from build123d import *

# Parameters (mm, degrees)
SKETCH_W           = 20
SKETCH_H           = 20
PAD_DEPTH          = 2
SKETCH001_W        = 21.291687
SKETCH001_H        = 2
PAD001_DEPTH       = 20
POCKET_DEPTH       = 43
PAD002_DEPTH       = 1
PAD003_DEPTH       = 1
SKETCH004_R        = 2.5
POCKET001_DEPTH    = 5
SKETCH005_R        = 2.5
POCKET002_DEPTH    = 5
POCKET003_DEPTH    = 5
POCKET003_FACE1_W  = 20
POCKET003_FACE1_H  = 2
POCKET004_DEPTH    = 1.846
POCKET005_DEPTH    = 2.202
POCKET006_DEPTH    = 5
SKETCH006_W        = 32.068451
SKETCH006_H        = 15.041733
POCKET007_DEPTH    = 5
POCKET008_DEPTH    = 2
POCKET009_DEPTH    = 2
POCKET010_DEPTH    = 0.5
POCKET011_DEPTH    = 0.5
POCKET011_FACE18_W = 2.5141439852
POCKET011_FACE18_H = 1
POCKET012_DEPTH    = 5
POCKET012_FACE12_W = 1
POCKET012_FACE12_H = 2.5
POCKET013_DEPTH    = 5
POCKET014_DEPTH    = 0.5
POCKET014_FACE5_W  = 1
POCKET014_FACE5_H  = 0.5
POCKET015_DEPTH    = 5
POCKET016_DEPTH    = 0.5
POCKET016_FACE4_W  = 0.5
POCKET016_FACE4_H  = 1
POCKET017_DEPTH    = 7.2
PAD004_DEPTH       = 3.202
PAD005_DEPTH       = 4.846


with BuildPart() as part:
    # Sketch → Pad (new body)
    with BuildSketch(Plane.XY):
        with Locations((318.7276667125, 240.4208782875)):
            Rectangle(SKETCH_W, SKETCH_H)
    extrude(amount=-PAD_DEPTH)

    # Sketch001 (on Face6 of Pad) → Pad001 (join)
    with BuildSketch(Plane(origin=(0, 0, -2), x_dir=(1, 0, 0), z_dir=(0, 0, -1))):
        with Locations((319.1250915, -231.419662)):
            Rectangle(SKETCH001_W, SKETCH001_H)
    extrude(amount=PAD001_DEPTH)

    # Pad001 Face5 → Pocket (cut)
    with BuildSketch(Plane(origin=(325.2175581813, 231.4103392408, -2), x_dir=(0, 1, 0), z_dir=(0, 0, 1))):
        Polygon((1.0093227592, 16.7383101813), (-0.9906772408, 16.7383101813), (-0.9906772408, -4.5533768187), (1.0093227592, -4.5533768187), (1.0093227592, -3.5101085312), (-0.9894609532, -3.5101085312), (-0.9894609532, 16.4898914688), (1.0093227592, 16.4898914688), align=None)
    extrude(amount=-POCKET_DEPTH, mode=Mode.SUBTRACT)

    # Sketch002 (on Face7 of Pocket) → Pad002 (join)
    with BuildSketch(Plane(origin=(308.7276667125, 0, 0), x_dir=(0, -1, 0), z_dir=(-1, 0, 0))):
        Polygon((-250.405853, 0), (-230.420715, -22), (-230.420715, 0), align=None)
    extrude(amount=-PAD002_DEPTH)

    # Sketch003 (on Face2 of Pad002) → Pad003 (join)
    with BuildSketch(Plane.YZ.offset(328.7276667125)):
        Polygon((230.420883, 0.034144), (250.420822, 0.034144), (230.420883, -22.000002), align=None)
    extrude(amount=-PAD003_DEPTH)

    # Sketch004 (on Face6 of Pad003) → Pocket001 (cut)
    with BuildSketch(Plane(origin=(0, 232.419662, 0), x_dir=(-1, 0, 0), z_dir=(0, 1, 0))):
        with Locations((-318.723811, -11.999702)):
            Circle(SKETCH004_R)
    extrude(amount=-POCKET001_DEPTH, mode=Mode.SUBTRACT)

    # Sketch005 (on Face5 of Pocket001) → Pocket002 (cut)
    with BuildSketch(Plane(origin=(0, 0, -2), x_dir=(1, 0, 0), z_dir=(0, 0, -1))):
        with Locations((318.727692, -240.420898)):
            Circle(SKETCH005_R)
    extrude(amount=-POCKET002_DEPTH, mode=Mode.SUBTRACT)

    # Pocket002 Face19 → Pocket003 (cut)
    with BuildSketch(Plane(origin=(327.7276667125, 240.4131065518, 0.0170764125), x_dir=(0, 1, 0), z_dir=(-1, 0, 0))):
        Polygon((-9.9922235518, -0.0170675875), (10.0077154482, -0.0170675875), (9.976723645, 0.0170764125), (-9.9922235518, 0.0170764125), align=None)
    extrude(amount=-POCKET003_DEPTH, mode=Mode.SUBTRACT)

    # Pocket003 Face1 → Pocket004 (cut)
    with BuildSketch(Plane(origin=(318.7276667125, 250.4208782875, -1), x_dir=(1, 0, 0), z_dir=(0, 1, 0))):
        Rectangle(POCKET003_FACE1_W, POCKET003_FACE1_H)
    extrude(amount=-POCKET004_DEPTH, mode=Mode.SUBTRACT)

    # Pocket004 Face7 → Pocket005 (cut)
    with BuildSketch(Plane(origin=(318.7276662811, 231.4202701891, -22), x_dir=(0, -1, 0), z_dir=(0, 0, -1))):
        Polygon((-0.9993918109, 9.9999995686), (-0.9993918109, -10.0000004314), (0.9993853738, -10.0000004314), (0.9993853738, -9.0000004314), (0.9993871891, -9.0000004314), (0.9993871891, -10.0000004314), (0.9993919016, -10.0000004314), (0.9993919016, 9.9999995686), align=None)
    extrude(amount=-POCKET005_DEPTH, mode=Mode.SUBTRACT)

    # Pocket005 Face11 → Pocket006 (cut)
    with BuildSketch(Plane(origin=(309.7276667125, 230.4207966437, -10.9999550626), x_dir=(0, -1, 0), z_dir=(1, 0, 0))):
        Polygon((-8.16439e-05, 10.9998651876), (-8.16439e-05, 8.7980449374), (-8.16439e-05, -10.9999550626), (8.16437e-05, -10.9999550626), (8.16437e-05, 11.0000449374), align=None)
    extrude(amount=-POCKET006_DEPTH, mode=Mode.SUBTRACT)

    # Sketch006 (on Face7 of Pocket006) → Pocket007 (cut)
    with BuildSketch(Plane(origin=(0, 0, -19.798), x_dir=(1, 0, 0), z_dir=(0, 0, -1))):
        with Locations((318.3954625, -232.1317065)):
            Rectangle(SKETCH006_W, SKETCH006_H)
    extrude(amount=POCKET007_DEPTH, mode=Mode.SUBTRACT)

    # Pocket007 Face15 → Pocket008 (cut)
    with BuildSketch(Plane(origin=(318.7273379116, 231.4203047573, -19.798), x_dir=(0, -1, 0), z_dir=(0, 0, -1))):
        Polygon((-0.9993572427, 8.9996711991), (-0.9993572427, -10.0003288009), (0.9994264698, -10.0003288009), (0.9994264698, 9.9996711991), (-1.0007408734, 9.9996711991), (-1.0007408734, 8.9996711991), align=None)
    extrude(amount=-POCKET008_DEPTH, mode=Mode.SUBTRACT)

    # Pocket008 Face3 → Pocket009 (cut)
    with BuildSketch(Plane(origin=(318.7276667125, 248.5748782875, -1), x_dir=(1, 0, 0), z_dir=(0, 1, 0))):
        Polygon((10, -1), (10, 1), (-9, 1), (-10, 1), (-10, -1), align=None)
    extrude(amount=-POCKET009_DEPTH, mode=Mode.SUBTRACT)

    # Pocket009 Face7 → Pocket010 (cut)
    with BuildSketch(Plane(origin=(318.7273379116, 231.4203047573, -17.798), x_dir=(0, -1, 0), z_dir=(0, 0, -1))):
        Polygon((-0.9993572427, 8.9996711991), (-0.9993572427, -9.0003288009), (-0.9993572427, -10.0003288009), (0.9994264698, -10.0003288009), (0.9994264698, 9.9996711991), (-1.0007408734, 9.9996711991), (-1.0007408734, 8.9996711991), align=None)
    extrude(amount=-POCKET010_DEPTH, mode=Mode.SUBTRACT)

    # Pocket010 Face3 → Pocket011 (cut)
    with BuildSketch(Plane(origin=(318.7276667125, 246.5748782875, -1), x_dir=(1, 0, 0), z_dir=(0, 1, 0))):
        Polygon((10, -1), (10, 1), (9, 1), (-9, 1), (-10, 1), (-10, -1), align=None)
    extrude(amount=-POCKET011_DEPTH, mode=Mode.SUBTRACT)

    # Pocket011 Face18 → Pocket012 (cut)
    with BuildSketch(Plane(origin=(309.2276667125, 247.3319502801, -2), x_dir=(0, 1, 0), z_dir=(0, 0, 1))):
        Rectangle(POCKET011_FACE18_W, POCKET011_FACE18_H)
    extrude(amount=-POCKET012_DEPTH, mode=Mode.SUBTRACT)

    # Pocket012 Face12 → Pocket013 (cut)
    with BuildSketch(Plane(origin=(309.2276667125, 232.4210456307, -18.548), x_dir=(-1, 0, 0), z_dir=(0, -1, 0))):
        Rectangle(POCKET012_FACE12_W, POCKET012_FACE12_H)
    extrude(amount=-POCKET013_DEPTH, mode=Mode.SUBTRACT)

    # Pocket013 Face14 → Pocket014 (cut)
    with BuildSketch(Plane(origin=(318.7269644137, 231.6380559444, -17.298), x_dir=(0, -1, 0), z_dir=(0, 0, -1))):
        Polygon((-3.0507371065, -10.0007022988), (1.2171776569, -10.0007022988), (1.2171776569, 9.9992977012), (-3.0540280954, 9.9992977012), (-3.0540280954, 8.9992977012), (-0.7816060556, 8.9992977012), (-0.7816060556, -9.0007022988), (-3.0507371065, -9.0007022988), align=None)
    extrude(amount=-POCKET014_DEPTH, mode=Mode.SUBTRACT)

    # Pocket014 Face5 → Pocket015 (cut)
    with BuildSketch(Plane(origin=(328.2276667125, 234.688793051, -17.048), x_dir=(-1, 0, 0), z_dir=(0, -1, 0))):
        Rectangle(POCKET014_FACE5_W, POCKET014_FACE5_H)
    extrude(amount=-POCKET015_DEPTH, mode=Mode.SUBTRACT)

    # Pocket015 Face3 → Pocket016 (cut)
    with BuildSketch(Plane(origin=(318.7247895723, 246.0748782875, -1.2887227346), x_dir=(1, 0, 0), z_dir=(0, 1, 0))):
        Polygon((10.0028771402, -1.2887227346), (10.0028771402, 3.4651057821), (9.0028771402, 3.4651057821), (9.0028771402, 0.7112772654), (-8.9971228598, 0.7112772654), (-8.9971228598, 3.4788922638), (-9.9971228598, 3.4788922638), (-9.9971228598, -1.2887227346), align=None)
    extrude(amount=-POCKET016_DEPTH, mode=Mode.SUBTRACT)

    # Pocket016 Face4 → Pocket017 (cut)
    with BuildSketch(Plane(origin=(328.2276667125, 245.8248782875, -4.7538285167), x_dir=(0, 1, 0), z_dir=(0, 0, 1))):
        Rectangle(POCKET016_FACE4_W, POCKET016_FACE4_H)
    extrude(amount=-POCKET017_DEPTH, mode=Mode.SUBTRACT)

    # Pocket017 Face4 → Pad004 (add)
    with BuildSketch(Plane(origin=(318.7269014881, 231.7036107724, -16.798), x_dir=(0, -1, 0), z_dir=(0, 0, -1))):
        Polygon((-3.4390219463, -10.0007652244), (1.2827324849, -10.0007652244), (1.2827324849, 9.9992347756), (-3.4426809492, 9.9992347756), (-3.4426809492, 8.9992347756), (-0.7160512276, 8.9992347756), (-0.7160512276, -9.0007652244), (-3.4390219463, -9.0007652244), align=None)
    extrude(amount=PAD004_DEPTH)

    # Pad004 Face2 → Pad005 (add)
    with BuildSketch(Plane(origin=(318.7249484764, 245.5748782875, -1.3772371444), x_dir=(1, 0, 0), z_dir=(0, 1, 0))):
        Polygon((10.002718236, -1.3772371444), (10.002718236, 3.9274467025), (9.002718236, 3.9274467025), (9.002718236, 0.6227628556), (-8.997281764, 0.6227628556), (-8.997281764, 3.940786863), (-9.997281764, 3.940786863), (-9.997281764, -1.3772371444), align=None)
    extrude(amount=PAD005_DEPTH)


solid = part.part
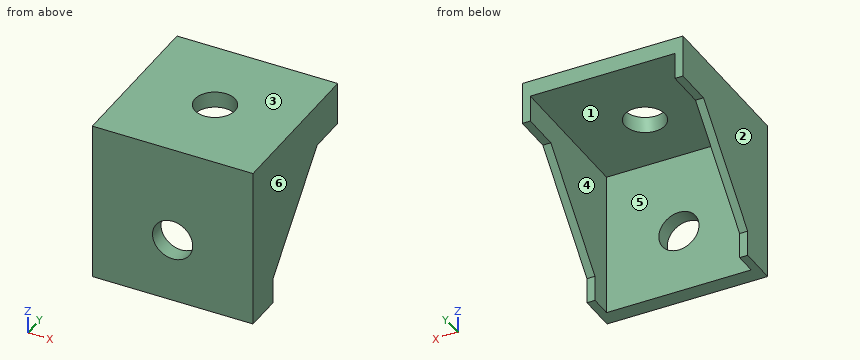
Here's how the part is built. I have some questions about the finished solid (model axes, mm). Face numbers are marked on the shaded views. A direction names the side the tool comes from. Coordinates: 2 decimals unless noted, no trailing zeros. Order: outer loops, then holes, each group sorted by start corner. A loop starts at its lowest first (then second) coordinate and runs counter-clockwise, first axis right, second up.
Item 1: For the marked faces 5 and 6, which set-ups out of +Z, -Z, +X, -X, +Y, -Y let a thin tool reach every point of the face, with its end or its side?
Result sheet:
face 5: -Z, +Y
face 6: +Z, -Z, +X, +Y, -Y
Item 2: For P1, Ø6, axis at x = 324, y = 242, coming from the -Z side; P2, Ø5.5, axis at x = 316, z = -15, coming from the +Y side; P3, Ø0.5, axis at x = 328.5, y = 247.5, coming from the -Z side, each with a flat end and sliding along its axis, tell me the tip position at first contact or that it passes through.
Result sheet:
P1: stops at z = -2
P2: stops at y = 232.42
P3: stops at z = -5.3
Item 3: If we section it at C-C on y = 239.25: List the corners of the cut face in (x, z) for me.
Result sheet:
outline: (308.73, -12.28) - (309.73, -12.28) - (309.73, -2) - (316.52, -2) - (316.52, 0) - (308.73, 0) - close; (320.94, -2) - (327.73, -2) - (327.73, -12.27) - (328.73, -12.27) - (328.73, 0) - (320.94, 0) - close
Item 4: I need wall thicknesses on line 1 (X direction, y = 239, z = -11.5); line 2 (Z direction, x = 327.25, y = 237.75); line 3 (Y direction, x = 311, z = -17.75). Which ranges of each line are inside material? Lowest first, please.
Result sheet:
line 1: x = 308.73 to 309.73, 327.73 to 328.73
line 2: z = -2 to 0
line 3: y = 230.42 to 232.42
Item 5: If we mould it in two halves opening along X, with no side actions, what happens to the marked faces 1, 2, 3 and 4? For each: +X half, -X half, draft (parallel to the pull), parting line (faces both ways), or undercut.
Result sheet:
face 1: undercut
face 2: -X half
face 3: draft
face 4: undercut
Item 6: If we section it at A-A on y = 233.5: List the corners of the cut face in (x, z) for me.
Result sheet:
outline: (308.73, -20) - (309.73, -20) - (309.73, -2) - (327.73, -2) - (327.73, -20) - (328.73, -20) - (328.73, 0) - (308.73, 0) - close
Item 7: If we section it at B-B on z = -13: List the corners of the cut face in (x, y) for me.
Result sheet:
outline: (308.73, 230.42) - (316.43, 230.42) - (316.43, 232.42) - (309.73, 232.42) - (309.73, 238.6) - (308.73, 238.6) - close; (321.01, 230.42) - (328.73, 230.42) - (328.73, 238.59) - (327.73, 238.59) - (327.73, 232.42) - (321.01, 232.42) - close
Item 8: If we section it at D-D on x = 317.5: List the corners of the cut face in (y, z) for me, plus the area to 3 significant figures.
Result sheet:
outline: (230.42, -20) - (232.42, -20) - (232.42, -14.18) - (230.42, -14.18) - close; (230.42, -9.82) - (232.42, -9.82) - (232.42, -2) - (238.24, -2) - (238.24, 0) - (230.42, 0) - close; (242.6, -2) - (250.42, -2) - (250.42, 0) - (242.6, 0) - close
area: 58.6 mm2
